Could you check a few things on this model? Use its own coordinates, in mm. Face numbers are marked on the shaded views. A direction names the side the tool comes from. Round coordinates to 2 decimals unless told otherwise and drop trailing zeros. Order: outer loops, then holes, each group sorted by start corner. A loop starts at its lowest first (then second) coordinate and runs counter-clockwise, first axis right, second up. Notation, with made-up numbers: M -17.75,-5.5 L 38.25,-5.5 A25 cw 38.25,10.5 Z; hole C 16.25,43.5 d3. An arc over 180 degrees is marked long. Write each question's results on one line, items separated by ' | '. Start each with the question number.
1. Suppose I cut it at C-C on x = 29. Write out the boundary of the cut face in (y, z).
2. Suppose I cut it at B-B on y = 47. Write out the boundary of the cut face in (x, z).
3. Suppose I cut it at D-D on y = 42.5. Write out the boundary of the cut face in (x, z), and give its area (3 significant figures).
4. Please list where these lines run through material, in increasing order: L1, parallel to X at y = 54.5, z = 8; L2, parallel to X at y = 50.5, z = 8.5; L3, parallel to Z at x = 42.5, y = 52.25.
5. I'm going to push flat-ended pins straight in: pin 1 (5 mm diameter, centred on x = 51.5, z = 4, fed in from -Y); pin 2 (10 mm diameter, centred on x = 35, y = 54, fed in from -Z); pin 3 (1.5 mm diameter, centred on x = 48, z = 4.5, fed in from +Y); pin 4 (6 mm diameter, centred on x = 14, y = 58, fed in from -Z). Where does each tip first touch, or does it pass through?
6. For the marked faces 5, 6, 7 and 8, which set-ups out of +Z, -Z, +X, -X, +Y, -Y let a thin tool reach every point of the face, with its end or its side?
7. We'd pull the mould along X, two halves only. Please class the marked faces 1, 2, 3 and 4: released by +X, released by -X, zero draft, split by the parting line, or undercut.
8. Suppose I cut it at A-A on z = 1.25. Give the number of separate pieces and of enclosed holes in the cut face, and give its area (3 significant figures).
Autodesk Inventor part; units mm, degrees
ref_plane "YZ Plane" through (0, 0, 0) normal (1, 0, 0) x (0, 1, 0)
ref_plane "XZ Plane" through (0, 0, 0) normal (0, 1, 0) x (-1, 0, 0)
ref_plane "XY Plane" through (0, 0, 0) normal (0, 0, 1) x (1, 0, 0)
sketch "Эскиз1" plane through (0, 0, 0) normal (0, 0, 1) x (1, 0, 0)
  circle A0 centre (33.0944, 52) radius 10
  circle A1 centre (53.0944, 52) radius 2
  circle A2 centre (13.0944, 52) radius 2
  line L0 (48.0944, 37) -> (18.0944, 37)
  line L1 (18.0944, 37) -> (18.0944, 67)
  line L2 (18.0944, 67) -> (48.0944, 67)
  line L3 (48.0944, 67) -> (48.0944, 37)
  line L4 (18.0944, 46) -> (7.0944, 46)
  line L5 (7.0944, 46) -> (7.0944, 58)
  line L6 (7.0944, 58) -> (18.0944, 58)
  line L7 (18.0944, 58) -> (18.0944, 46)
  line L8 (48.0944, 46) -> (60.0944, 46)
  line L9 (60.0944, 46) -> (60.0944, 58)
  line L10 (60.0944, 58) -> (48.0944, 58)
  line L11 (48.0944, 58) -> (48.0944, 46)
  point P0 (0, 0)
  dimension "d0" = 15
  dimension "d1" = 15
  dimension "d2" = 15
  dimension "d3" = 15
  dimension "d4" = 6
  dimension "d5" = 6
  dimension "d6" = 6
  dimension "d7" = 12
  dimension "d8" = 12
extrude "Выдавливание1" add sketch "Эскиз1" along normal blind 4
fillet "Сопряжение1" radius 15 4 edges at (18.0944, 37, 2) (18.0944, 67, 2) (48.0944, 37, 2) (48.0944, 67, 2)
fillet "Сопряжение2" radius 6 4 edges at (60.0944, 58, 2) (60.0944, 46, 2) (7.0944, 46, 2) (7.0944, 58, 2)
sketch "Эскиз2" plane through (0, 0, 4) normal (0, 0, 1) x (1, 0, 0)
  circle A0 centre (33.0944, 52) radius 10
  circle A1 centre (33.0944, 52) radius 8.75
  circle A2 centre (33.0944, 52) radius 10
  circle A3 centre (53.0944, 52) radius 2
  circle A4 centre (13.0944, 52) radius 2
  arc A5 (13.0944, 58) -> (13.0944, 46) centre (13.0944, 52) ccw
  line L0 (13.0944, 46) -> (18.0944, 46)
  arc A6 (18.0944, 46) -> (31.8421, 37) centre (31.8421, 52) ccw
  line L1 (31.8421, 37) -> (34.3467, 37)
  arc A7 (34.3467, 37) -> (48.0944, 46) centre (34.3467, 52) ccw
  line L2 (48.0944, 46) -> (54.0944, 46)
  arc A8 (54.0944, 46) -> (54.0944, 58) centre (54.0944, 52) ccw
  line L3 (54.0944, 58) -> (48.0944, 58)
  arc A9 (48.0944, 58) -> (34.3467, 67) centre (34.3467, 52) ccw
  line L4 (34.3467, 67) -> (31.8421, 67)
  arc A10 (31.8421, 67) -> (18.0944, 58) centre (31.8421, 52) ccw
  line L5 (18.0944, 58) -> (13.0944, 58)
  point P0 (0, 0)
  dimension "d13" = 17.5
extrude "Выдавливание2" add sketch "Эскиз2" along normal blind 5 contours A0 | L5 A10 L4 A9 L3 A8 L2 A7 L1 A6 L0 A5
sketch "Эскиз3" plane through (0, 0, 9) normal (0, 0, 1) x (1, 0, 0)
  circle A0 centre (33.0944, 52) radius 8.75
  circle A1 centre (13.0944, 52) radius 2
  circle A2 centre (53.0944, 52) radius 2
  arc A3 (13.0944, 58) -> (13.0944, 46) centre (13.0944, 52) ccw
  line L0 (13.0944, 46) -> (18.0944, 46)
  arc A4 (18.0944, 46) -> (31.8421, 37) centre (31.8421, 52) ccw
  line L1 (31.8421, 37) -> (34.3467, 37)
  arc A5 (34.3467, 37) -> (48.0944, 46) centre (34.3467, 52) ccw
  line L2 (48.0944, 46) -> (54.0944, 46)
  arc A6 (54.0944, 46) -> (54.0944, 58) centre (54.0944, 52) ccw
  line L3 (54.0944, 58) -> (48.0944, 58)
  arc A7 (48.0944, 58) -> (34.3467, 67) centre (34.3467, 52) ccw
  line L4 (34.3467, 67) -> (31.8421, 67)
  arc A8 (31.8421, 67) -> (18.0944, 58) centre (31.8421, 52) ccw
  line L5 (18.0944, 58) -> (13.0944, 58)
  circle A9 centre (33.0944, 52) radius 7
  point P0 (0, 0)
  dimension "d16" = 14
extrude "Выдавливание3" add sketch "Эскиз3" along normal blind 2 contours A0 | L5 A8 L4 A7 L3 A6 L2 A5 L1 A4 L0 A3
sketch "Эскиз4" plane through (0, 0, 11) normal (0, 0, 1) x (1, 0, 0)
  circle A0 centre (13.0944, 52) radius 2
  circle A1 centre (53.0944, 52) radius 2
  line L0 (9.4717, 49.6281) -> (9.2289, 53.9514)
  line L1 (9.2289, 53.9514) -> (12.8516, 56.3233)
  line L2 (12.8516, 56.3233) -> (16.7171, 54.3719)
  line L3 (16.7171, 54.3719) -> (16.9599, 50.0486)
  line L4 (16.9599, 50.0486) -> (13.3372, 47.6767)
  line L5 (13.3372, 47.6767) -> (9.4717, 49.6281)
  line L6 (50.591, 48.4669) -> (48.7829, 52.4014)
  line L7 (48.7829, 52.4014) -> (51.2863, 55.9346)
  line L8 (51.2863, 55.9346) -> (55.5978, 55.5331)
  line L9 (55.5978, 55.5331) -> (57.4059, 51.5986)
  line L10 (57.4059, 51.5986) -> (54.9025, 48.0654)
  line L11 (54.9025, 48.0654) -> (50.591, 48.4669)
  point P0 (0, 0)
  dimension "d19" = 7.5
  dimension "d20" = 7.5
extrude "Выдавливание4" cut sketch "Эскиз4" against normal blind 4
equation "\"d20\" = d19"
properties part number "ппрофиль"
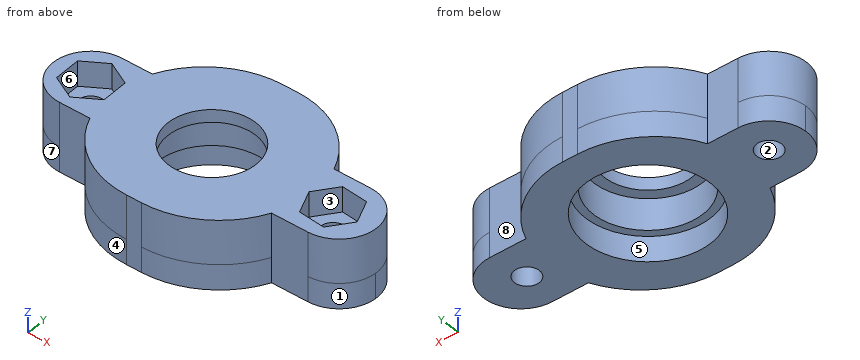
Filled sheet:
1) outline: M 37.27,0 L 42.88,0 L 42.88,4 L 44.27,4 L 44.27,9 L 46.32,9 L 46.32,11 L 37.27,11 Z; M 57.68,9 L 59.73,9 L 59.73,4 L 61.12,4 L 61.12,0 L 66.73,0 L 66.73,11 L 57.68,11 Z
2) outline: M 9.78,0 L 24.43,0 L 24.43,4 L 25.91,4 L 25.91,9 L 28.2,9 L 28.2,11 L 9.78,11 Z; M 37.99,9 L 40.28,9 L 40.28,4 L 41.75,4 L 41.75,0 L 57.41,0 L 57.41,11 L 37.99,11 Z
3) outline: M 20.23,0 L 29.97,0 L 29.97,4 L 36.22,4 L 36.22,0 L 45.95,0 L 45.95,11 L 20.23,11 Z | area: 258 mm^2
4) L1: x = 7.64 to 10.07, 16.46 to 24.71, 41.48 to 50.27, 56.07 to 59.55 | L2: x = 7.28 to 9.42, 16.93 to 24.47, 41.71 to 49.66, 56.63 to 59.9 | L3: z = 4 to 11
5) pin 1: stops at y = 46 | pin 2: stops at z = 9 | pin 3: stops at y = 59.65 | pin 4: stops at z = 0
6) face 5: -Z | face 6: +Z | face 7: +Z, -Z, -X, -Y | face 8: +Z, -Z, +X, +Y
7) face 1: released by +X | face 2: undercut | face 3: undercut | face 4: released by -X
8) separate pieces: 1 | enclosed holes: 3 | area: 668 mm^2
